The figure shows three views and two pictorial views of one solid part (mm, origin at its lowest corner). Answer the questions. A direction names the side the tool comes from. Coordinates: 2 decimals unless noted, no trailing zeros. Order: outer loops, then holes, each group sorted by start corner. A loop starts at its lowest first (then second) coordinate and runs counter-clockwise, first axis right, second up. Notation, with made-up numbers: (37, -33) -> (67, -33) arc R22 cw to (67, -2) -> close; hole circle Ø10 at (52.25, -14). An arc over 180 degrees is marked (long way). Return JSON: item names as keys, results as strings.
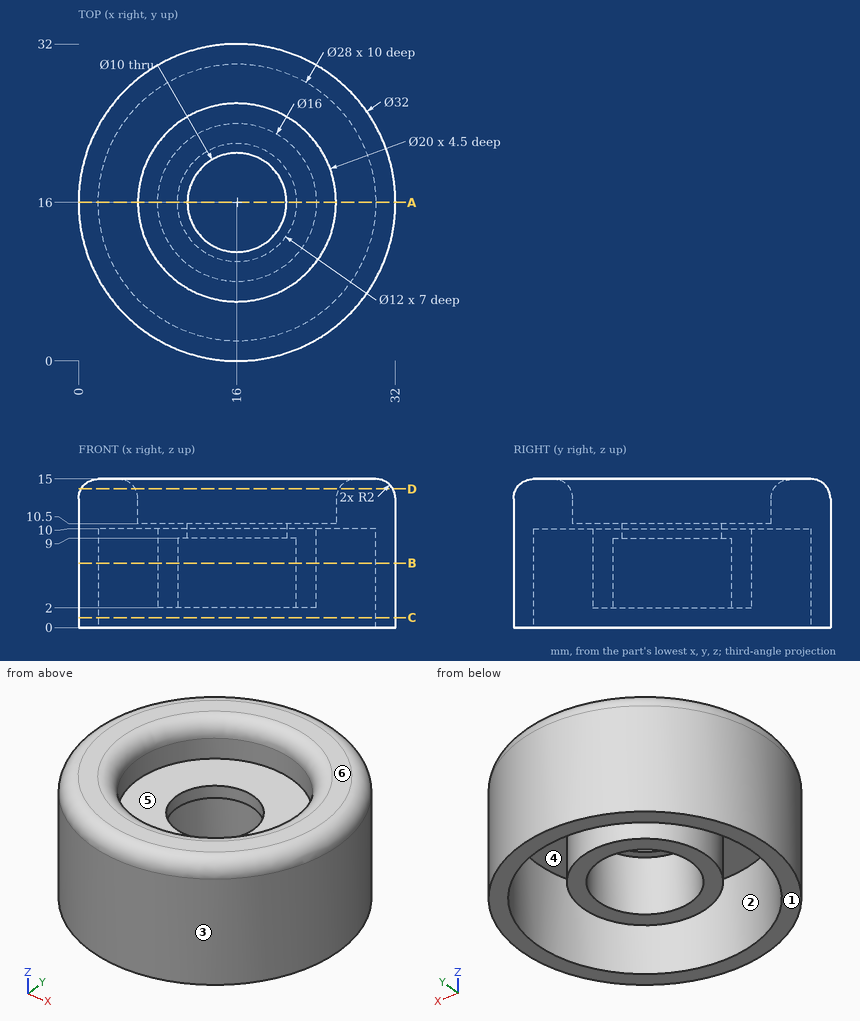
1. The part is cut by section D-D on z = 14. Give the vertices of the cut face in (x, y).
Answer block:
{"outline": "circle Ø31.46 at (16, 16); hole circle Ø20.54 at (16, 16)"}
2. Each of these flat-tipped pins is pushed along its axis until it touches: pin 1 Ø9.5 at (x, y) = (16, 17) entering from -Z; pin 2 Ø5 at (x, y) = (14.5, 16.5) entering from -Z; pin 3 Ø6 at (x, z) = (21, 5.5) entering from -Y; pin 4 Ø3 at (y, z) = (4.5, 2.5) entering from +X. Where does it stop, or does it pass through?
Answer block:
{"pin 1": "stops at z = 9", "pin 2": "passes through", "pin 3": "stops at y = 0.13", "pin 4": "stops at x = 28.49"}
3. The part is cut by section A-A on y = 16. Give the vertices of the cut face in (x, z), and give its area (3 significant figures).
Answer block:
{"outline": "(0, 0) -> (2, 0) -> (2, 10) -> (8, 10) -> (8, 2) -> (10, 2) -> (10, 9) -> (11, 9) -> (11, 10.5) -> (6, 10.5) -> (6, 13) arc R2 ccw to (4, 15) -> (2, 15) arc R2 ccw to (0, 13) -> close; (21, 9) -> (22, 9) -> (22, 2) -> (24, 2) -> (24, 10) -> (30, 10) -> (30, 0) -> (32, 0) -> (32, 13) arc R2 ccw to (30, 15) -> (28, 15) arc R2 ccw to (26, 13) -> (26, 10.5) -> (21, 10.5) -> close", "area": "136 mm2"}
4. For the marked faces 4, 5 and 6, determine the directions among +Z, -Z, +X, -X, +Y, -Y from which every point of the face is accessible in a straight line to the end or side of a thin tool.
Answer block:
{"face 4": "-Z", "face 5": "+Z", "face 6": "+Z, +X, -X, +Y, -Y"}
5. Determine the mould class of the marked faces 1, 2 and 3 for opening direction Y: pulls with the +Y half, pulls with the -Y half, needs draft (parallel to the pull), parting line crosses it, or undercut.
Answer block:
{"face 1": "needs draft", "face 2": "undercut", "face 3": "parting line crosses it"}
6. Consider line 1 (Y direction, x = 16, z = 9.7); line 2 (Y direction, x = 16, z = 4); line 3 (Y direction, x = 16, z = 12.25). Determine where each line is inside the solid, lowest interval first. Write a range as from..to.
Answer block:
{"line 1": "y = 0..2, 8..11, 21..24, 30..32", "line 2": "y = 0..2, 8..10, 22..24, 30..32", "line 3": "y = 0..6, 26..32"}
7. The part is cut by section B-B on z = 6.5. Give the vertices of the cut face in (x, y), and give its area (3 significant figures).
Answer block:
{"outline": "circle Ø32 at (16, 16); circle Ø16 at (16, 16); hole circle Ø28 at (16, 16); hole circle Ø12 at (16, 16)", "area": "276 mm2"}
8. The part is cut by section C-C on z = 1. Give the vertices of the cut face in (x, y), and give its area (3 significant figures).
Answer block:
{"outline": "circle Ø32 at (16, 16); hole circle Ø28 at (16, 16)", "area": "188 mm2"}
